The model under review builds one solid part; all positions refer to its coordinate system, in mm. A direction names the side the tool comes from. Coordinates: 2 decimals unless noted, no trailing zeros. Loops run counter-clockwise (first coordinate to the right, second up) from the corner with the lowest first, then second, coordinate; pieces in that order, holes last. Notation, with made-up numbers: M 85,66.5 L 141,66.5 A23 ccw 141,88.5 Z; hole C 48.5,52.25 d2. An arc over 180 degrees is marked long. Return JSON: item names as keys, results as strings.
Autodesk Inventor part; units mm, degrees
ref_plane "YZ Plane" through (0, 0, 0) normal (1, 0, 0) x (0, 1, 0)
ref_plane "XZ Plane" through (0, 0, 0) normal (0, 1, 0) x (-1, 0, 0)
ref_plane "XY Plane" through (0, 0, 0) normal (0, 0, 1) x (1, 0, 0)
sketch "Sketch1" plane through (0, 0, 0) normal (0, 1, 0) x (-1, 0, 0)
  line L0 (16.2222, 35.2121) -> (-14.7778, 35.2121)
  line L1 (-14.7778, 35.2121) -> (-14.7778, -34.7879)
  line L2 (-14.7778, -34.7879) -> (16.2222, -34.7879)
  line L3 (16.2222, -34.7879) -> (16.2222, 35.2121)
  point P0 (0, 0)
  dimension "d0" = 70
  dimension "d1" = 31
extrude "Extrusion1" add sketch "Sketch1" along normal blind 60
sketch "Sketch3" plane through (14.7778, 0, 35.2121) normal (1, 0, 0) x (0, 0, -1)
  circle A0 centre (35.2121, 35.5368) radius 27.5
  point P0 (35.2121, 0)
  dimension "d5" = 55
hole "Hole1" at (14.7778, 35.5368, 0) direction (-1, 0, 0) diameter 55 end through all
sketch "Sketch6" plane through (0, 60, 0) normal (0, 1, 0) x (1, 0, 0)
  line L0 (-0.0667, -13.4045) -> (-0.0667, 12.7365)
  line L1 (-16.2222, 0) -> (14.7778, 0) construction
  circle A0 centre (-0.0667, -12.8895) radius 4
  circle A1 centre (-0.0667, 12.5336) radius 4
  point P0 (0, 0)
  point P1 (14.7778, -12.562)
  point P2 (-16.2222, -12.562)
  point P3 (-16.2222, 12.562)
  point P4 (14.7778, 12.562)
  dimension "d42" = 8
  dimension "d43" = 8
sketch "Sketch8" plane through (0, 60, 0) normal (0, 1, 0) x (1, 0, 0)
  line L0 (14.7778, 34.7879) -> (-16.2222, 34.7879) construction
  line L1 (-16.2222, 0) -> (14.7778, 0) construction
  circle A0 centre (5, -28) radius 2
  circle A1 centre (5, 28) radius 2
  point P0 (0, 0)
  dimension "d33" = 4
extrude "Extrusion4" cut sketch "Sketch6" against normal blind 4
sketch "Sketch15" plane through (0, 60, 0) normal (0, 1, 0) x (1, 0, 0)
  arc A0 (-4.0532, -12.562) -> (3.9199, -12.562) centre (-0.0667, -12.8895) ccw
  line L0 (-0.0667, -16.8895) -> (14.7778, -16.8895)
  line L1 (14.7778, 27.5) -> (14.7778, -27.5)
  line L2 (14.7778, -12.562) -> (14.7778, -16.8895)
  line L3 (14.7778, -12.562) -> (3.9199, -12.562)
  line L4 (-0.0667, -12.8895) -> (-0.0667, -12.8895)
  arc A1 (3.9332, 12.562) -> (-4.0666, 12.562) centre (-0.0667, 12.5336) ccw
  line L5 (-0.0667, 16.5336) -> (-0.0667, 12.5336)
  line L6 (3.9332, 12.562) -> (14.7778, 12.562)
  line L7 (14.7778, 12.562) -> (14.7778, 16.5336)
  line L8 (14.7778, 16.5336) -> (-0.0667, 16.5336)
  line L9 (-0.0667, -12.562) -> (14.7778, -12.562)
  line L10 (-0.0667, -12.562) -> (-0.0667, -16.8895)
  line L11 (14.7778, 12.562) -> (-0.0667, 12.5336)
  point P0 (0, 0)
extrude "Extrusion5" cut sketch "Sketch15" against normal blind 4 contours A0 L3 L1 L0 | L1 L6 A1 L8
hole "Hole5" at (5, 60, 28) at (5, 60, -28) direction (0, -1, 0) diameter 5 depth 14
sketch "Sketch18" plane through (0, 0, 0) normal (0, -1, 0) x (1, 0, 0)
  line L0 (-16.2222, -34.7879) -> (-63.2222, -34.7879)
  line L1 (-16.2222, 35.2121) -> (-63.2222, 35.2121)
  line L2 (-63.2222, 35.2121) -> (-63.2222, -34.7879)
  line L3 (-16.2222, -34.7879) -> (-16.2222, 35.2121)
  line L4 (-63.2222, -34.7879) -> (-63.2222, 35.2121)
  point P0 (0, 0)
  dimension "d57" = 47
extrude "Extrusion9" add sketch "Sketch18" against normal blind 2
sketch "Sketch25" plane through (0, 0, 0) normal (0, -1, 0) x (1, 0, 0)
  line L0 (-63.2222, 35.2121) -> (14.7778, 35.2121)
  line L1 (14.7778, 35.2121) -> (14.7778, -34.7879)
  line L2 (14.7778, -34.7879) -> (-63.2222, -34.7879)
  line L3 (-63.2222, -34.7879) -> (-63.2222, 35.2121)
  point P0 (0, 0)
extrude "Extrusion11" add sketch "Sketch25" along normal blind 5
sketch "Sketch29" plane through (0, 2, 0) normal (0, 1, 0) x (1, 0, 0)
  point P0 (0, 0)
sketch "Sketch37" plane through (0, 2, 0) normal (0, 1, 0) x (1, 0, 0)
  point P0 (0, 0)
sketch "Sketch39" plane through (0, 2, 0) normal (0, 1, 0) x (1, 0, 0)
  line L0 (-16.2222, -35.2121) -> (-41.2222, -35.2121)
  line L1 (-41.2222, -35.2121) -> (-41.2222, -12.2121)
  line L2 (-41.2222, -12.2121) -> (-16.2222, -12.2121)
  line L3 (-16.2222, -12.2121) -> (-16.2222, -35.2121)
  point P0 (0, 0)
  dimension "d120" = 25
  dimension "d121" = 23
extrude "Extrusion27" add sketch "Sketch39" along normal blind 122
sketch "Sketch43" plane through (0, 2, 0) normal (0, 1, 0) x (1, 0, 0)
  line L0 (-16.2222, 34.7879) -> (-63.2222, 34.7879)
  line L1 (-41.2222, -35.2121) -> (-44.39, -35.2121)
  line L2 (-44.39, -35.2121) -> (-44.39, 34.7879)
  line L3 (-44.39, 34.7879) -> (-41.2222, 34.7879)
  line L4 (-41.2222, 34.7879) -> (-41.2222, -35.2121)
  point P0 (0, 0)
extrude "Extrusion28" add sketch "Sketch43" along normal blind 53.526
properties part number "BF_base_model"
1. The part is to be moulded in two halves that separate along Z. For faces 1 (the face through (7, 59, 16.89)), 2 (the face through (-29, 62, 12.212)), 3 (the face through (-16.222, 20, -24)), say which applies: released by +Z, released by -Z, zero draft, split by the parting line, or undercut.
Check values:
{"face 1": "undercut", "face 2": "released by -Z", "face 3": "zero draft"}
2. To check wall thickness, follow line 1 (X direction, y = 49.5, z = -28); line 2 (X direction, y = 49, z = 28); line 3 (Z direction, x = 5, y = 52). State the ranges of each line that lie inside material, in increasing order.
Check values:
{"line 1": "-44.39 to -41.22, -16.22 to 2.5, 7.5 to 14.78", "line 2": "-44.39 to 2.5, 7.5 to 14.78", "line 3": "-34.79 to -30.5, -25.5 to -22.03, 22.03 to 25.5, 30.5 to 35.21"}
3. Machinability: for faces 4 (the face through (-1, 60, 24)), 5 (the face through (-44.39, 28, 1)), 6 (the face through (5, 46, 28)), which of the approach directions +Z, -Z, +X, -X, +Y, -Y give a long, thin tool a straight path to every point of the face, cutting with its end or side? Answer none if there is none.
Check values:
{"face 4": "+Z, -Z, +X, +Y", "face 5": "+Z, -Z, -X, +Y", "face 6": "+Y"}
4. Add section D-D on x = 5. Give the boundary of the cut face in (y, z).
Check values:
{"outline": "M -5,-34.79 L 60,-34.79 L 60,-30.5 L 46,-30.5 L 46,-25.5 L 60,-25.5 L 60,-16.53 L 57.51,-16.53 A27.5 cw long 57.24,16.89 L 60,16.89 L 60,25.5 L 46,25.5 L 46,30.5 L 60,30.5 L 60,35.21 L -5,35.21 Z"}
5. Add section A-A on y = 53. Give the boundary of the cut face in (x, z), plus the area to 3 significant figures.
Check values:
{"outline": "M -44.39,-34.79 L -41.22,-34.79 L -41.22,12.21 L -16.22,12.21 L -16.22,21.24 L 14.78,21.24 L 14.78,35.21 L -44.39,35.21 Z; M -16.22,-34.79 L 14.78,-34.79 L 14.78,-21.24 L -16.22,-21.24 Z; hole C 5,-28 d5; hole C 5,28 d5", "area": "1,610 mm²"}
6. Insertion check: pin 1 Ø1.5 at (x, z) = (-35.5, -6) entering from +Y; pin 2 Ø8 at (x, z) = (5, 28) entering from +Y; pin 3 Ø8 at (y, z) = (33.5, 22.5) entering from +X; pin 4 Ø12 at (y, z) = (55.5, -16.5) entering from +X. Each pin has a flat end and moves straight along its axis. Give the tip position at first contact, or say it passes through.
Check values:
{"pin 1": "y = 2", "pin 2": "y = 60", "pin 3": "x = -16.22", "pin 4": "x = 14.78"}
7. Add section B-B on y = 30. Give the boundary of the cut face in (x, z).
Check values:
{"outline": "M -44.39,-34.79 L -41.22,-34.79 L -41.22,12.21 L -16.22,12.21 L -16.22,26.94 L 14.78,26.94 L 14.78,35.21 L -44.39,35.21 Z; M -16.22,-34.79 L 14.78,-34.79 L 14.78,-26.94 L -16.22,-26.94 Z"}
8. Add section C-C on z = -24. Give the boundary of the cut face in (x, y).
Check values:
{"outline": "M -63.22,-5 L 14.78,-5 L 14.78,22.11 L -16.22,22.11 L -16.22,2 L -41.22,2 L -41.22,55.53 L -44.39,55.53 L -44.39,2 L -63.22,2 Z; M -16.22,48.96 L 14.78,48.96 L 14.78,60 L -16.22,60 Z"}
